from build123d import *

# Parameters (mm, degrees)
ESQUISSE1_R             = 13
BOSS_EXTRU_1_DEPTH      = 12
BOSS_EXTRU_2_START      = -12
ESQUISSE2_R             = 13
ESQUISSE2_R_2           = 5.5
BOSS_EXTRU_2_DEPTH      = 3
ESQUISSE4_R             = 8
ENL_V_MAT_EXTRU_2_DEPTH = 6
ESQUISSE5_R             = 3
ENL_V_MAT_EXTRU_3_DEPTH = 69.271516755
ESQUISSE6_W             = 10
ESQUISSE6_H             = 6
ENL_V_MAT_EXTRU_4_DEPTH = 12
CHANFREIN1_SIZE         = 5
ESQUISSE7_R             = 1
ENL_V_MAT_EXTRU_5_DEPTH = 12


with BuildPart() as part:
    # Esquisse1 → Boss.-Extru.1 (new body)
    with BuildSketch(Plane.XY):
        Polygon((-40, 0), (40, 0), (40, 25), (17, 25), (17, 55), (-17, 55), (-17, 25), (-40, 25), align=None)
        with Locations((0, 40)):
            Circle(ESQUISSE1_R, mode=Mode.SUBTRACT)
    extrude(amount=BOSS_EXTRU_1_DEPTH)

    # Esquisse2 → Boss.-Extru.2 (add)
    with BuildSketch(Plane.XY.offset(12).offset(BOSS_EXTRU_2_START)):
        with Locations((0, 40)):
            Circle(ESQUISSE2_R)
        with Locations((0, 40)):
            Circle(ESQUISSE2_R_2, mode=Mode.SUBTRACT)
    extrude(amount=BOSS_EXTRU_2_DEPTH)

    # Esquisse4 → Enlèv. mat.-Extru.2 (cut)
    with BuildSketch(Plane(origin=(0, 0, 0), x_dir=(-1, 0, 0), z_dir=(0, 0, -1))):
        with Locations((-25, 15)):
            Circle(ESQUISSE4_R)
        with Locations(Location((25, 15, 0), (0, 0, 180))):
            Circle(ESQUISSE4_R)
    extrude(amount=-ENL_V_MAT_EXTRU_2_DEPTH, mode=Mode.SUBTRACT)

    # Esquisse5 → Enlèv. mat.-Extru.3 (cut, through all)
    with BuildSketch(Plane(origin=(0, 0, 6), x_dir=(-1, 0, 0), z_dir=(0, 0, -1))):
        with Locations((-25, 15)):
            Circle(ESQUISSE5_R)
        with Locations(Location((25, 15, 0), (0, 0, 180))):
            Circle(ESQUISSE5_R)
    extrude(amount=-ENL_V_MAT_EXTRU_3_DEPTH, mode=Mode.SUBTRACT)

    # Esquisse6 → Enlèv. mat.-Extru.4 (cut)
    with BuildSketch(Plane.XY.offset(12)):
        with Locations((35, 3)):
            Rectangle(ESQUISSE6_W, ESQUISSE6_H)
        with Locations((-35, 3)):
            Rectangle(ESQUISSE6_W, ESQUISSE6_H)
    extrude(amount=-ENL_V_MAT_EXTRU_4_DEPTH, mode=Mode.SUBTRACT)

    # Chanfrein1
    chanfrein1_edges = [part.edges().sort_by_distance(p)[0] for p in [
        (-17, 55, 6),
        (17, 55, 6),
        (17, 25, 6),
        (40, 25, 6),
        (-40, 25, 6),
        (-17, 25, 6),
    ]]
    chamfer(chanfrein1_edges, length=CHANFREIN1_SIZE)

    # Esquisse7 → Enlèv. mat.-Extru.5 (cut)
    with BuildSketch(Plane(origin=(0, 0, 0), x_dir=(-1, 0, 0), z_dir=(0, 0, -1))):
        with Locations((-10, 45)):
            Circle(ESQUISSE7_R)
        with Locations(Location((10, 45, 0), (0, 0, 180))):
            Circle(ESQUISSE7_R)
        with Locations((-37, 15)):
            Circle(ESQUISSE7_R)
        with Locations(Location((37, 15, 0), (0, 0, 180))):
            Circle(ESQUISSE7_R)
        with Locations((0, 15)):
            Circle(ESQUISSE7_R)
    extrude(amount=-ENL_V_MAT_EXTRU_5_DEPTH, mode=Mode.SUBTRACT)


solid = part.part
Geometry: final body of the model. Coordinates: model frame, mm. A direction names the side the tool comes from. Give positions to 0.01 mm unless a question says otherwise; leave off trailing zeros. Loops run counter-clockwise (first coordinate to the right, second up) from the corner with the lowest first, then second, coordinate; pieces in that order, holes last. Notation, with made-up numbers: M 61,-29.75 L 107,-29.75 A21 ccw 107,-22.75 Z; hole C -0.75,-37 d11. An arc over 180 degrees is marked long. Put each result on its own line as item: value. Start each with the question number.
1) Contact query for flat-ended pins moving along their axis: pin 1 (5 mm diameter, centred on x = 21, y = 16.5, fed in from -Z); pin 2 (3.5 mm diameter, centred on x = 25, y = 15, fed in from -Z); pin 3 (4 mm diameter, centred on y = 36.5, z = 6.5, fed in from +X); pin 4 (6.5 mm diameter, centred on y = 2, z = 5.5, fed in from +X). Output: stop coordinate, or through.
2) Ray query, line 1 along Y through (x, z) = (0, 0.7); line 2 along Y through (x, z) = (0, 10.5); line 3 along X through (y, z) = (13.5, 7.25). Return the intervals inside material, ascending.
3) Cut plane A-A (y = 15). Give the number of separate pieces and of enclosed holes in the cut face, then the cut area to 3 significant figures.
4) Cut plane B-B (x = 0). Output: boundary loops of the cut face in (y, z), then the cut area to 3 significant figures.
5) Pull-direction query (Y, two-part tool) for faces 5 (the flat face through (17, 40, 6)), 6 (the cylindrical face through (10, 46, 1)), 7 (the flat face through (0, 0, 6)); classes: pulls with the +Y half, pulls with the -Y half, needs draft (parallel to the pull), parting line crosses it, or undercut.
6) Access query for faces 1 (the flat face through (30, 3, 6)), 2 (the cylindrical face through (26.73, 7.19, 2.96)), 3 (the flat face through (6, 40, 3)), 4 (the flat face through (29, 25, 6)). Directions: +Z, -Z, +X, -X, +Y, -Y. A direction counts if a zero-diameter tool reaches every point of the face in a straight line with its end or side. Return the directions, or none.
7) Cut plane D-D (z = 8). Output: boundary loops of the cut face in (x, y).
8) Cut plane C-C (x = -37). Output: boundary loops of the cut face in (y, z).
Verdict:
1. pin 1: z = 6
1. pin 2: through
1. pin 3: x = 17
1. pin 4: x = 30
2. line 1: 0 to 14, 16 to 34.5, 45.5 to 55
2. line 2: 0 to 14, 16 to 27, 53 to 55
2. line 3: -40 to -27.6, -22.4 to 22.4, 27.6 to 40
3. separate pieces: 6
3. enclosed holes: 0
3. area: 624 mm2
4. outline: M 0,0 L 14,0 L 14,12 L 0,12 Z; M 16,0 L 34.5,0 L 34.5,3 L 27,3 L 27,12 L 16,12 Z; M 45.5,0 L 55,0 L 55,12 L 53,12 L 53,3 L 45.5,3 Z
4. area: 369 mm2
5. face 5: needs draft
5. face 6: undercut
5. face 7: pulls with the -Y half
6. face 1: +Z, -Z, +X, -Y
6. face 2: -Z
6. face 3: +Z
6. face 4: +Z, -Z, +X, +Y
7. outline: M -40,6 L -30,6 L -30,0 L 30,0 L 30,6 L 40,6 L 40,20 L 35,25 L 22,25 L 17,30 L 17,50 L 12,55 L -12,55 L -17,50 L -17,30 L -22,25 L -35,25 L -40,20 Z; hole C -37,15 d2; hole C -25,15 d6; hole C 0,40 d26; hole C 0,15 d2; hole C 25,15 d6; hole C 37,15 d2
8. outline: M 6,0 L 14,0 L 14,12 L 6,12 Z; M 16,0 L 23,0 L 23,12 L 16,12 Z
